Geometry: see drawing. Coordinates: mm, zero at the bounding-box minimum. A direction names the side the tool comes from. Coordinates: 2 decimals unless noted, no trailing zeros. Loops run counter-clockwise (first coordinate to the right, second up) from the corner with the lowest first, then second, coordinate; pieces in that order, holes last. Notation, with made-up numbers: (85, 19) - (137, 19) arc R18 ccw to (137, 36) - close; hole circle Ø8 at (-3, 36). An arc over 180 degrees is marked (long way). Use a Markdown table: item, result. Add a question column.
1. Section query C-C on x = 15. Return the cut outline in (y, z).
2. Section query A-A on y = 45. Return the cut outline in (x, z), then the cut area to 3 significant figures.
3. Access query for the marked faces 1 and 2. Directions: +Z, -Z, +X, -X, +Y, -Y. A direction counts if a zero-diameter tool reaches every point of the face in a straight line with its end or side. Return the directions, or none.
4. Draft query along Z for the marked faces 3, 4 and 5. Return one class per face: released by +Z, released by -Z, zero draft, split by the parting line, or undercut.
5. Section query D-D on y = 56. Return the cut outline in (x, z), then the cut area to 3 significant figures.
6. Ray query, L1, parallel to Y at x = 12.5, z = 13.5; L2, parallel to X at y = 38.5, z = 10.5; L3, parallel to Z at x = 15, y = 59. Return the intervals inside material, ascending. Write a range as [from, to].
7. Section query B-B on z = 10. Return the cut outline in (x, y).
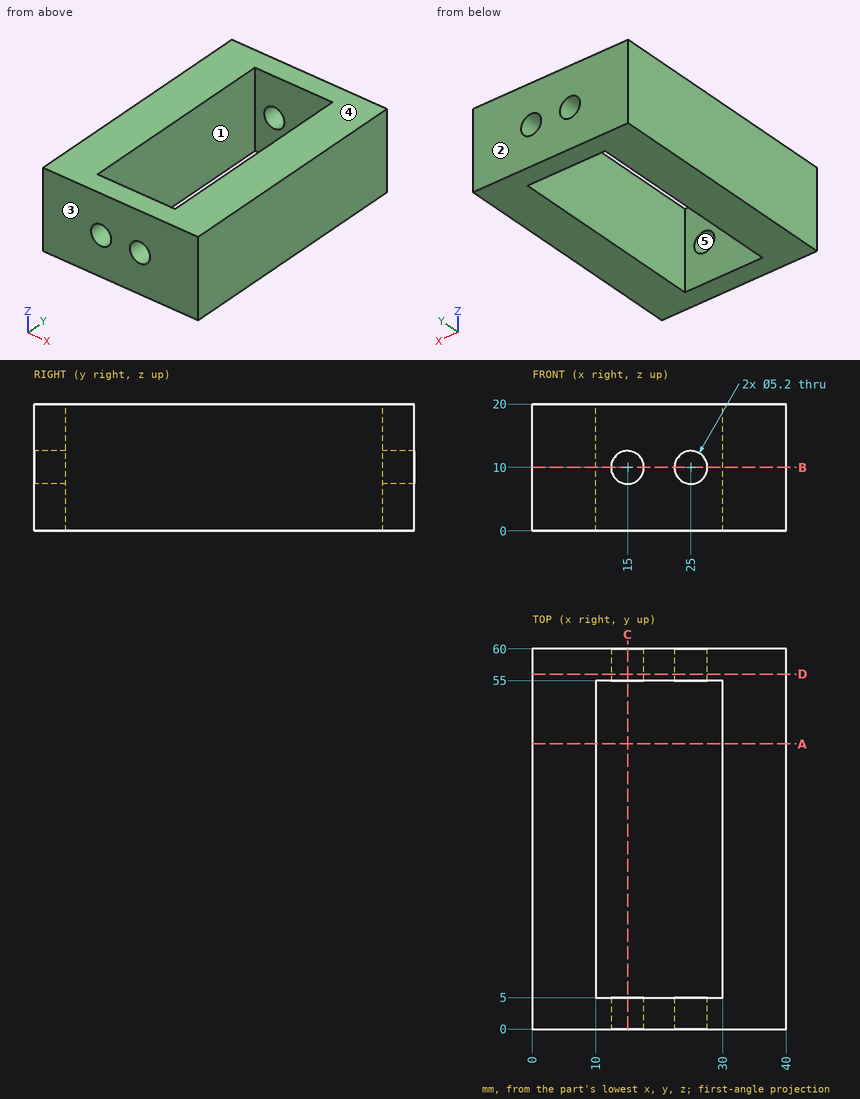
Resolved:
| question | item | result |
|---|---|---|
| 1 | outline | (0, 0) - (5, 0) - (5, 7.4) - (0, 7.4) - close; (0, 12.6) - (5, 12.6) - (5, 20) - (0, 20) - close; (55, 0) - (60, 0) - (60, 7.4) - (55, 7.4) - close; (55, 12.6) - (60, 12.6) - (60, 20) - (55, 20) - close |
| 2 | outline | (0, 0) - (10, 0) - (10, 20) - (0, 20) - close; (30, 0) - (40, 0) - (40, 20) - (30, 20) - close |
| 2 | area | 400 mm² |
| 3 | face 1 | +Z, -Z |
| 3 | face 2 | +Z, -Z, +X, -X, +Y |
| 4 | face 3 | zero draft |
| 4 | face 4 | released by +Z |
| 4 | face 5 | undercut |
| 5 | outline | (0, 0) - (40, 0) - (40, 20) - (0, 20) - close; hole circle Ø5.2 at (15, 10); hole circle Ø5.2 at (25, 10) |
| 5 | area | 758 mm² |
| 6 | L1 | [0, 5], [55, 60] |
| 6 | L2 | [0, 10], [30, 40] |
| 6 | L3 | [0, 7.4], [12.6, 20] |
| 7 | outline | (0, 0) - (12.4, 0) - (12.4, 5) - (10, 5) - (10, 55) - (12.4, 55) - (12.4, 60) - (0, 60) - close; (17.6, 0) - (22.4, 0) - (22.4, 5) - (17.6, 5) - close; (17.6, 55) - (22.4, 55) - (22.4, 60) - (17.6, 60) - close; (27.6, 0) - (40, 0) - (40, 60) - (27.6, 60) - (27.6, 55) - (30, 55) - (30, 5) - (27.6, 5) - close |
